from build123d import *

# Parameters (mm, degrees)
F_3_4_16_TAPPED_HOLE1_D     = 17.4625
F_3_4_16_TAPPED_HOLE1_DEPTH = 20
F_3_4_16_TAPPED_HOLE1_TIP   = 5.24626428
CUT_EXTRUDE1_REACH          = 95.91
SKETCH5_R                   = 7.5


with BuildPart() as part:
    # Sketch1 → Revolve1 (revolve)
    with BuildSketch(Plane(origin=(0, 0, 0), x_dir=(0, 0, -1), z_dir=(1, 0, 0))):
        Polygon((0, 27), (12.7, 27), (12.7, 7), (25, 7), (25, 0), (15.68, 0), (10.16, -20.600920458), (10.16, -60), (0, -60), align=None)
    revolve(axis=Axis((0, 0, 0), (0, 1, 0)))

    # 3/4-16 Tapped Hole1
    with Locations(Plane(origin=(0, 27, 0), x_dir=(1, 0, 0), z_dir=(0, 1, 0))):
        with Locations((0, 0)):
            Hole(F_3_4_16_TAPPED_HOLE1_D / 2, depth=F_3_4_16_TAPPED_HOLE1_DEPTH)
            with Locations((0, 0, -(F_3_4_16_TAPPED_HOLE1_DEPTH + F_3_4_16_TAPPED_HOLE1_TIP / 2))):  # 118° drill point
                Cone(0, F_3_4_16_TAPPED_HOLE1_D / 2, F_3_4_16_TAPPED_HOLE1_TIP, mode=Mode.SUBTRACT)

    # Cut-Extrude1: up to this cone (the profile starts outside it)
    cut_extrude1_end = Plane(origin=(0, -60, 0), z_dir=(0, 1, 0)).offset(61.75373672) * Cone(1.664e-06, 57.677709576, 34.65626328, align=(Align.CENTER, Align.CENTER, Align.MIN), mode=Mode.PRIVATE)
    # Sketch5 → Cut-Extrude1 (cut, up to the surface)
    with BuildSketch(Plane.XZ.offset(60), mode=Mode.PRIVATE) as cut_extrude1_sk1:
        with Locations(Location((0, 0, 0), (0, 0, 270))):
            Circle(SKETCH5_R)
    cut_extrude1_tool1 = extrude(cut_extrude1_sk1.sketch, amount=-CUT_EXTRUDE1_REACH, mode=Mode.PRIVATE) - cut_extrude1_end
    add(cut_extrude1_tool1.solids().sort_by_distance((0, -60, 0))[0], mode=Mode.SUBTRACT)


solid = part.part
Build history of the part. All positions in model axes, mm. A direction names the side the tool comes from. Coordinates: 2 decimals unless noted, no trailing zeros. Order: outer loops, then holes, each group sorted by start corner. A loop starts at its lowest first (then second) coordinate and runs counter-clockwise, first axis right, second up. Notation, with made-up numbers: (87, -28.75) - (110, -28.75) arc R23 ccw to (110, -12.75) - close; hole circle Ø8 at (0, -26.5). An arc over 180 degrees is marked (long way). Write item = value, one per line. Start each with the question number.
1) Saw through at C-C on y = 4. Write the cut outline in (x, z), then the cut area to 3 significant figures.
2) Saw through at D-D on z = 20. Write the cut outline in (x, y).
3) 3-axis set-ups, long thin cutter, end or side, ignore diameter. For faces 4 (the face through (-10.074, -40.576, 1.323)), 5 (the face through (-7.509, 3.451, -23.846)), 6 (the face through (-5.9, 7, -11.5)): which of +Z, -Z, +X, -X, +Y, -Y reach the whole face in a straight line?
4) Two-plate mould, pull along X, no slides. Class faces 1 (the face through (12.4, 16.86, 2.75)), 2 (the face through (6.93, 16.86, 5.31)), 3 (the face through (-9, 27, 3)): pulls with the +X half, pulls with the -X half, needs draft (parallel to the pull), parting line crosses it, or undercut.
5) Saw through at A-A on x = 0. Write the cut outline in (y, z), then the cut area to 3 significant figures.
6) Flat gauge pins, fed straight in: pin 1 Ø10 at (y, z) = (-41, 19) entering from +X; pin 2 Ø6 at (x, y) = (-12, -50) entering from +Z; pin 3 Ø20 at (x, z) = (0, 0) entering from +Y; pin 4 Ø17 at (x, z) = (0, 0) entering from +Y. Where does each tip first touch, or does it go through?
7) Saw through at B-B on z = 0. Write the cut outline in (x, y).
8) Wall check: line 1 along Z through (x, y) = (0, -22.5); line 2 along Y through (x, z) = (14.5, -16). Give the ranges that are in metal, low to high. Write a range as from..to.
From the geometry:
q1.outline = circle Ø50 at (0, 0); hole circle Ø15 at (0, 0)
q1.area = 1,790 mm^2
q2.outline = (-15, 0) - (15, 0) - (15, 7) - (-15, 7) - close
q3.face_4 = -Y
q3.face_5 = +Y, -Y
q3.face_6 = +Y
q4.face_1 = parting line crosses it
q4.face_2 = undercut
q4.face_3 = needs draft
q5.outline = (-60, -10.16) - (-20.6, -10.16) - (0, -15.68) - (0, -25) - (7, -25) - (7, -12.7) - (27, -12.7) - (27, -8.73) - (7, -8.73) - (6.26, -7.5) - (-60, -7.5) - close; (-60, 7.5) - (6.26, 7.5) - (7, 8.73) - (27, 8.73) - (27, 12.7) - (7, 12.7) - (7, 25) - (0, 25) - (0, 15.68) - (-20.6, 10.16) - (-60, 10.16) - close
q5.area = 836 mm^2
q6.pin_1 = through
q6.pin_2 = 4.71
q6.pin_3 = 27
q6.pin_4 = 6.86
q7.outline = (-25, 0) - (-15.68, 0) - (-10.16, -20.6) - (-10.16, -60) - (-7.5, -60) - (-7.5, 6.26) - (-8.73, 7) - (-8.73, 27) - (-12.7, 27) - (-12.7, 7) - (-25, 7) - close; (7.5, -60) - (10.16, -60) - (10.16, -20.6) - (15.68, 0) - (25, 0) - (25, 7) - (12.7, 7) - (12.7, 27) - (8.73, 27) - (8.73, 7) - (7.5, 6.26) - close
q8.line_1 = -10.16..-7.5, 7.5..10.16
q8.line_2 = 0..7
